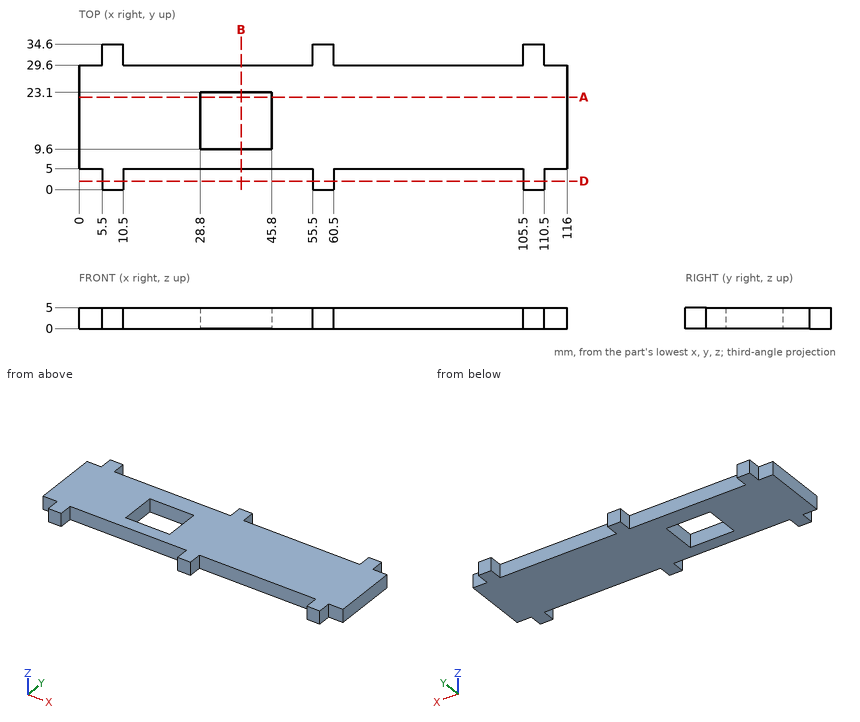
The drawing under review shows one solid part. Ordinate dimensions are in mm from its lowest x, y, z. Coordinates: 2 decimals unless noted, no trailing zeros. Write each loop counter-clockwise with the first axis right and the second up, starting at its lowest first coordinate (ties: lowest second). Pieces come first, ordered by that corner, then holes. Notation, with made-up numbers: (87, 3.5) - (143, 3.5) arc R18 cw to (143, 13.5) - close; hole circle Ø9 at (83.25, 24). An arc over 180 degrees is marked (long way). Answer in a Markdown table with one row per item. Add a question column.
Q1. We need section A-A, the plane y = 22. State the section outline as (x, z) points.
Q2. For P1, Ø2.5, axis at y = 32.5, z = 3.5, coming from the +X side; P2, Ø2.5, axis at x = 114, z = 1.5, coming from the +Y side; P3, Ø1.5, axis at y = 32.5, z = 1.5, coming from the -X side; P4, Ø1, axis at y = 28.5, z = 3.5, coming from the -X side, all flat-tipped, find the tip position at first contact; note any pin that passes through.
Q3. We need section B-B, the plane x = 38.5. State the section outline as (y, z) points.
Q4. We need section D-D, the plane y = 2. State the section outline as (x, z) points, and give its area (3 significant figures).
Q5. For probe 1 along X at (y, z) = (30.5, 4.1); probe 2 along X at (y, z) = (17, 3.8); probe 3 along Y at (x, z) = (34.5, 1.9), list the stretches that pass through material, from the lowest coordinate up.
Answer list:
| question | item | result |
|---|---|---|
| 1 | outline | (0, 0) - (28.8, 0) - (28.8, 5) - (0, 5) - close; (45.8, 0) - (116, 0) - (116, 5) - (45.8, 5) - close |
| 2 | P1 | stops at x = 110.5 |
| 2 | P2 | stops at y = 29.6 |
| 2 | P3 | stops at x = 5.5 |
| 2 | P4 | stops at x = 0 |
| 3 | outline | (5, 0) - (9.6, 0) - (9.6, 5) - (5, 5) - close; (23.1, 0) - (29.6, 0) - (29.6, 5) - (23.1, 5) - close |
| 4 | outline | (5.5, 0) - (10.5, 0) - (10.5, 5) - (5.5, 5) - close; (55.5, 0) - (60.5, 0) - (60.5, 5) - (55.5, 5) - close; (105.5, 0) - (110.5, 0) - (110.5, 5) - (105.5, 5) - close |
| 4 | area | 75.0 mm2 |
| 5 | probe 1 | x = 5.5 to 10.5, 55.5 to 60.5, 105.5 to 110.5 |
| 5 | probe 2 | x = 0 to 28.8, 45.8 to 116 |
| 5 | probe 3 | y = 5 to 9.6, 23.1 to 29.6 |
